Solid Edge part; units mm, degrees
sketch "Sketch1" plane through (0, 0, 0) normal (0, 0, 1) x (1, 0, 0)
  circle A0 centre (0, 0) radius 7.3
  circle A1 centre (0, 0) radius 4.3
extrude "Protrusion1" add sketch "Sketch1" along normal blind 42
chamfer "Chamfer_1" distance 1 angle 45 1 edges at (-4.3, 0, 42)
sketch "Sketch2" plane through (0, 0, 0) normal (0, 0, -1) x (0, -1, 0)
  line L0 (-8, -8) -> (8, -8)
  line L1 (8, -8) -> (8, 8)
  line L2 (8, 8) -> (-8, 8)
  line L3 (-8, 8) -> (-8, -8)
  dimension "D1" = 8
  dimension "D2" = 8
extrude "ExtrudedProtrusion_4" add sketch "Sketch2" along normal blind 6
Check sheet for the modelled part. Datum: model origin and axes. Units: mm. A direction names the side the tool comes from. Give positions to 0.01 mm unless a question says otherwise; leave off trailing zeros. Write each loop counter-clockwise with the first axis right and the second up, starting at its lowest first coordinate (ties: lowest second). Pieces come first, ordered by that corner, then holes. Notation, with made-up numbers: (39.5, -29.5) - (53.5, -29.5) arc R33 cw to (53.5, 1.5) - close; hole circle Ø7 at (37, 83.25). An arc over 180 degrees is marked (long way). Answer as a JSON object with one key per item and string values. Group by question number.
1) Access from +Z, -Z, +X, -X, +Y, -Y to the whole of each face (thin tool, end or side, straight path). Record for faces 5 (the face through (2.4, -7.1, 0)), 6 (the face through (-8, 0, -3)).
2) Depth check by flat-ended pin: P1, Ø2, axis at x = -5, z = 23, coming from the +Y side; P2, Ø4, axis at x = -2.5, z = 5, coming from the -Y side; P3, Ø2, axis at x = 2.5, y = 1.5, coming from the +Z side. Enter the tip coordinate at first touch or a pass-through.
3) Sectioned sample at C-C (z = 32). Record the cut outline in (x, y).
4) Sectioned sample at A-A (x = 0). Record the cut outline in (y, z).
5) Thickness scan on probe 1 along Y at (x, z) = (0, 27); probe 2 along Z at (x, y) = (5.75, -5.5); probe 3 along X at (y, z) = (1, 7.5). Record the ranges inside material, lowest first. Write a range as from..to.
6) Sectioned sample at D-D (x = -6.25). Record the cut outline in (y, z).
7) Release check for a two-part mould opening along Y. For faces 1 (the face through (0, -8, -3)), 2 (the face through (-4.296, -0.189, 20.213)), 3 (the face through (0, 0, 0)), 4 (the face through (4, 4, 42)) record: pulls with the +Y half, pulls with the -Y half, needs draft (parallel to the pull), parting line crosses it, or undercut.
Geometry results:
{
 "1": {"face 5": "+Z", "face 6": "+Z, -Z, -X, +Y, -Y"},
 "2": {"P1": "stops at y = 6.11", "P2": "stops at y = -7.28", "P3": "stops at z = 0"},
 "3": {"outline": "circle Ø14.6 at (0, 0); hole circle Ø8.6 at (0, 0)"},
 "4": {"outline": "(-8, -6) - (8, -6) - (8, 0) - (7.3, 0) - (7.3, 42) - (5.3, 42) - (4.3, 41) - (4.3, 0) - (-4.3, 0) - (-4.3, 41) - (-5.3, 42) - (-7.3, 42) - (-7.3, 0) - (-8, 0) - close"},
 "5": {"probe 1": "y = -7.3..-4.3, 4.3..7.3", "probe 2": "z = -6..0", "probe 3": "x = -7.23..-4.18, 4.18..7.23"},
 "6": {"outline": "(-8, -6) - (8, -6) - (8, 0) - (3.77, 0) - (3.77, 42) - (-3.77, 42) - (-3.77, 0) - (-8, 0) - close"},
 "7": {"face 1": "pulls with the -Y half", "face 2": "undercut", "face 3": "undercut", "face 4": "needs draft"}
}
